from build123d import *

# Parameters (mm, degrees)
FILLET1_R = 1.651


with BuildPart() as part:
    # Sketch1 → Revolve1 (revolve)
    with BuildSketch(Plane.XY):
        Polygon((34.1757, 0), (34.1757, 12.7), (38.1, 12.7), (38.1, 8.509), (35.56, 8.509), (35.56, 4.699), (38.1, 4.699), (38.1, 0), align=None)
    revolve(axis=Axis((0, 13.335, 0), (0, -1, 0)))

    # Fillet1
    fillet1_edges = [part.edges().sort_by_distance(p)[0] for p in [
        (-35.56, 4.699, 0),
        (-35.56, 8.509, 0),
    ]]
    fillet(fillet1_edges, radius=FILLET1_R)


solid = part.part
Design review of the part built by this model. Coordinates are the model's own, in mm. A direction names the side the tool comes from. Round coordinates to 2 decimals unless told otherwise and drop trailing zeros. Write each loop counter-clockwise with the first axis right and the second up, starting at its lowest first coordinate (ties: lowest second). Pieces come first, ordered by that corner, then holes.
Item 1: Draft analysis for pull direction Y (two halves, no side actions). For faces 3 (the cylindrical face through (-7.709, 6.6, -34.714)), 4 (the flat face through (-14.29, 0, 31.22)), 5 (the flat face through (-8, 4.699, -37)), 6 (the flat face through (14.29, 12.7, 31.22)), state which applies: released by +Y, released by -Y, zero draft, split by the parting line, or undercut.
Item 2: Consider section A-A on z = 0. Give the boundary of the cut face in (x, y).
Item 3: Consider section B-B on x = 0. Give the boundary of the cut face in (y, z), and give its area (3 significant figures).
Item 4: Wall thickness on L1, parallel to Z at x = 0, y = 3.5; L2, parallel to X at y = 6.25, z = 1; L3, parallel to Z at x = 0, y = 6.5: over which ranges is each line inside the solid? List them lowest first.
Item 5: Consider section C-C on y = 1. Give the boundary of the cut face in (x, z).
Item 6: For pin 1 Ø6 at (y, z) = (9, 6.5) entering from -X; pin 2 Ø5 at (x, y) = (-23, 6.5) entering from +Z; pin 3 Ø2 at (y, z) = (11.5, 11) entering from +X, all flat-tipped, find the tip position at first contact; note any pin that passes through.
Item 7: For faces 1 (the cylindrical face through (-30.235, 10.575, -23.183)), 2 (the flat face through (8, 8.509, -37)), list the 3-axis set-ups (+Z, -Z, +X, -X, +Y, -Y) from which the entire face can be reached by the end or side of a thin tool; tool diameter is ignored.
Check values:
1. face 3: undercut
1. face 4: released by -Y
1. face 5: undercut
1. face 6: released by +Y
2. outline: (-38.1, 0) - (-34.18, 0) - (-34.18, 12.7) - (-38.1, 12.7) - (-38.1, 8.51) - (-37.21, 8.51) arc R1.65 cw to (-35.56, 6.86) - (-35.56, 6.35) arc R1.65 cw to (-37.21, 4.7) - (-38.1, 4.7) - close; (34.18, 0) - (38.1, 0) - (38.1, 4.7) - (37.21, 4.7) arc R1.65 cw to (35.56, 6.35) - (35.56, 6.86) arc R1.65 cw to (37.21, 8.51) - (38.1, 8.51) - (38.1, 12.7) - (34.18, 12.7) - close
3. outline: (0, -38.1) - (4.7, -38.1) - (4.7, -37.21) arc R1.65 cw to (6.35, -35.56) - (6.86, -35.56) arc R1.65 cw to (8.51, -37.21) - (8.51, -38.1) - (12.7, -38.1) - (12.7, -34.18) - (0, -34.18) - close; (0, 34.18) - (12.7, 34.18) - (12.7, 38.1) - (8.51, 38.1) - (8.51, 37.21) arc R1.65 cw to (6.86, 35.56) - (6.35, 35.56) arc R1.65 cw to (4.7, 37.21) - (4.7, 38.1) - (0, 38.1) - close
3. area: 82.7 mm2
4. L1: z = -38.1 to -34.18, 34.18 to 38.1
4. L2: x = -35.55 to -34.16, 34.16 to 35.55
4. L3: z = -35.56 to -34.18, 34.18 to 35.56
5. outline: circle Ø76.2 at (0, 0); hole circle Ø68.35 at (0, 0)
6. pin 1: stops at x = -37.94
6. pin 2: stops at z = 31.61
6. pin 3: stops at x = 36.76
7. face 1: +Y, -Y
7. face 2: none
